Input: part model. Units: mm. Frame: model coordinates. A direction names the side the tool comes from. Round coordinates to 2 decimals unless told otherwise and drop trailing zeros. Loops run counter-clockwise (first coordinate to the right, second up) from the corner with the lowest first, then second, coordinate; pieces in that order, holes last.
1) Access query for faces 5 (the face through (6, 27, 3)), 6 (the face through (-2, 26, 3)), 7 (the face through (-6, 27, 3)), 8 (the face through (4, 21, 6)). Directions: +Z, -Z, +X, -X, +Y, -Y. A direction counts if a zero-diameter tool reaches every point of the face in a straight line with its end or side. Return the directions, or none.
2) Ray query, line 1 along X through (y, z) = (0, 1.25); line 2 along Y through (x, z) = (0, 4.3); line 3 along X through (y, z) = (7, 5.3) (3 decimals). Return the intervals inside material, ascending.
3) Draft query along Y for faces 1 (the face through (-2.6, 31.32, 3.04)), 2 (the face through (2, 26, 3)), 3 (the face through (-2.45, 20.37, 3.04)), 4 (the face through (2.475, 20.339, 3.042)). Return one class per face: pulls with the +Y half, pulls with the -Y half, needs draft (parallel to the pull), parting line crosses it, or undercut.
4) Section A-A, the plane y = 0. Return loops of the section in (x, z).
5) Section C-C, the plane x = -8.5. Return loops of the section in (y, z), and give its area (3 significant figures).
6) Section D-D, the plane x = 0. Return loops of the section in (y, z), and give its area (3 significant figures).
7) First-contact query: pin 1 (1.5 mm diameter, centred on x = 2, z = 2, fed in from -Y); pin 2 (2.5 mm diameter, centred on y = 27.5, z = 3.5, fed in from -X); pin 3 (1.5 mm diameter, centred on y = 19, z = 5, fed in from -X). Flat tips, straight axial feed; report the tip coordinate or a pass-through.
from build123d import *

# Parameters (mm, degrees)
BOSS_EXTRUDE1_DEPTH = 6
FILLET1_R           = 2


with BuildPart() as part:
    # Sketch1 → Boss-Extrude1 (new body)
    with BuildSketch(Plane.XY):
        with BuildLine():
            Line((-6, 23.237900077), (-6, 31.891873593))
            Line((-6, 31.891873593), (-2, 31.891873593))
            Line((-2, 31.891873593), (-2, 19.899748742))
            ThreePointArc((-2, 19.899748742), (0, -20), (2, 19.899748742))
            Line((2, 19.899748742), (2, 31.891873593))
            Line((2, 31.891873593), (6, 31.891873593))
            Line((6, 31.891873593), (6, 23.237900077))
            ThreePointArc((6, 23.237900077), (0, -24), (-6, 23.237900077))
        make_face()
    extrude(amount=BOSS_EXTRUDE1_DEPTH)

    # Fillet1
    fillet1_edges = [part.edges().sort_by_distance(p)[0] for p in [
        (-2, 19.899748742, 3),
        (2, 19.899748742, 3),
        (6, 23.237900077, 3),
        (-6, 23.237900077, 3),
        (6, 31.891873593, 3),
        (2, 31.891873593, 3),
        (-2, 31.891873593, 3),
        (-6, 31.891873593, 3),
    ]]
    fillet(fillet1_edges, radius=FILLET1_R - 0.0001)  # a hair under: the kernel refuses the full size


solid = part.part
Final values:
1. face 5: +Z, -Z, +X, +Y
1. face 6: +Z, -Z, +Y
1. face 7: +Z, -Z, -X, +Y
1. face 8: +Z, +X, -X, +Y, -Y
2. line 1: x = -24 to -20, 20 to 24
2. line 2: y = -24 to -20
2. line 3: x = -22.956 to -18.735, 18.735 to 22.956
3. face 1: pulls with the +Y half
3. face 2: needs draft
3. face 3: undercut
3. face 4: undercut
4. outline: (-24, 0) - (-20, 0) - (-20, 6) - (-24, 6) - close; (20, 0) - (24, 0) - (24, 6) - (20, 6) - close
5. outline: (-22.44, 0) - (-18.1, 0) - (-18.1, 6) - (-22.44, 6) - close; (18.1, 0) - (22.44, 0) - (22.44, 6) - (18.1, 6) - close
5. area: 52.1 mm2
6. outline: (-24, 0) - (-20, 0) - (-20, 6) - (-24, 6) - close
6. area: 24.0 mm2
7. pin 1: stops at y = -23.97
7. pin 2: stops at x = -6
7. pin 3: stops at x = -15.59
